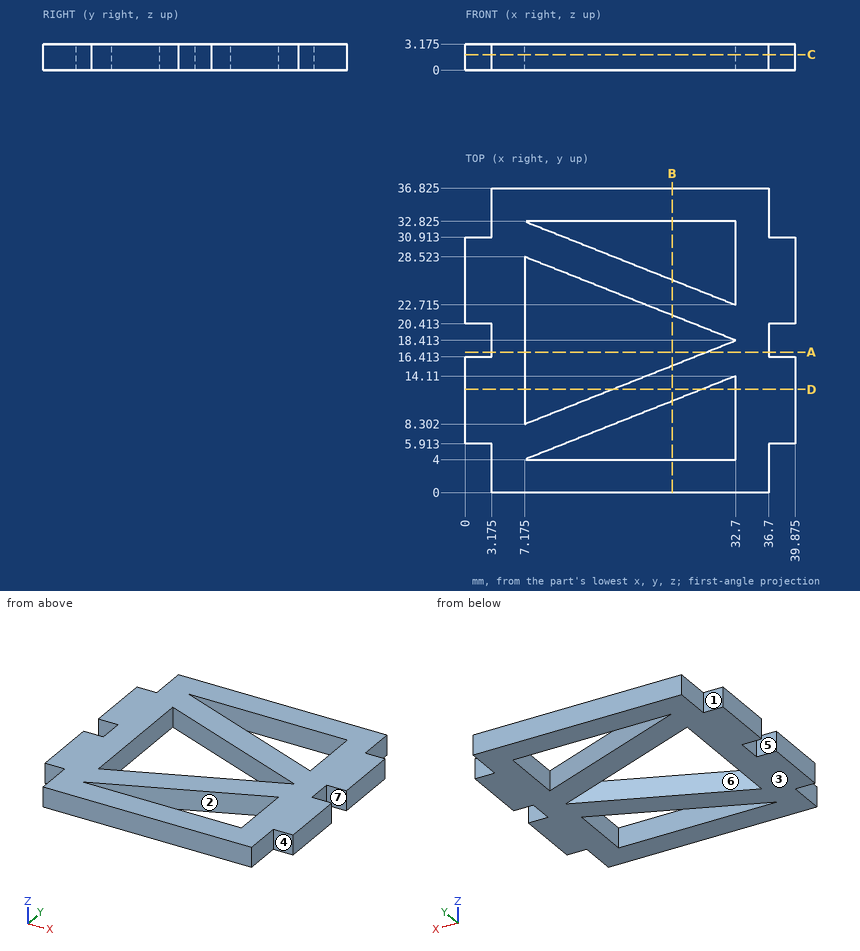
Design review of the part shown in the three views and the two pictorial views. Dimensions are in mm from the part's minimum x, y and z. A direction names the side the tool comes from. Give positions to 0.01 mm unless a question says otherwise; leave off trailing zeros. Loops run counter-clockwise (first coordinate to the right, second up) from the corner with the lowest first, then second, coordinate; pieces in that order, holes last. Notation, with made-up numbers: (1.25, -25) - (42.25, -25) arc R24 ccw to (42.25, -2) - close; hole circle Ø2 at (-22, 11). An arc over 180 degrees is marked (long way). Use CSV: the item, a comma, the result in double quotes. Start each with the question number.
1. Machinability: for the marked faces 4, 5, 6 and 7, which of the approach directions +Z, -Z, +X, -X, +Y, -Y give a long, thin tool a straight path to every point of the face, cutting with its end or side? Answer none if there is none.
2. Add section C-C (z = 1.9). Count the separate pieces of the cut face and the enclosed holes in it.
3. Draft analysis for pull direction Y (two halves, no side actions). For the marked faces 1, 2 and 3, state which applies: released by +Y, released by -Y, zero draft, split by the parting line, or undercut.
4. Add section D-D (y = 12.5). State the section outline as (x, z) points (1 decimal).
5. Wall thickness on L1, parallel to Y at x = 38, z = 1.7; L2, parallel to Y at x = 10, z = 0.4 (1 decimal); L3, parallel to Y at x = 17, z = 1.35 (1 decimal): over which ranges is each line inside the solid? List them lowest first.
6. Insertion check: P1, Ø1.6, axis at x = 38, z = 1, coming from the +Y side; P2, Ø1, axis at x = 1.5, z = 1, coming from the -Y side; P3, Ø1, axis at y = 4, z = 2.5, coming from the +X side. Each pin has a flat end and moves straight along its axis. Give the tip position at first contact, or say it passes through.
7. Add section B-B (x = 25). State the section outline as (y, z) points (1 decimal).
8. Add section A-A (y = 17). State the section outline as (x, z) points (1 decimal).
Results found:
1,face 4,"+Z, -Z, +X, -Y"
1,face 5,"+Z, -Z, -X"
1,face 6,"+Z, -Z"
1,face 7,"+Z, -Z, +X"
2,separate pieces,"1"
2,enclosed holes,"3"
3,face 1,"released by +Y"
3,face 2,"undercut"
3,face 3,"zero draft"
4,outline,"(0, 0) - (7.2, 0) - (7.2, 3.2) - (0, 3.2) - close; (17.8, 0) - (28.6, 0) - (28.6, 3.2) - (17.8, 3.2) - close; (32.7, 0) - (39.9, 0) - (39.9, 3.2) - (32.7, 3.2) - close"
5,L1,"y = 5.91 to 16.41, 20.41 to 30.91"
5,L2,"y = 0 to 4, 5.1 to 9.4, 27.4 to 31.7, 32.8 to 36.8"
5,L3,"y = 0 to 4, 7.9 to 12.2, 24.6 to 28.9, 32.8 to 36.8"
6,P1,"stops at y = 30.91"
6,P2,"stops at y = 5.91"
6,P3,"stops at x = 36.7"
7,outline,"(0, 0) - (4, 0) - (4, 3.2) - (0, 3.2) - close; (11.1, 0) - (15.4, 0) - (15.4, 3.2) - (11.1, 3.2) - close; (21.5, 0) - (25.8, 0) - (25.8, 3.2) - (21.5, 3.2) - close; (32.8, 0) - (36.8, 0) - (36.8, 3.2) - (32.8, 3.2) - close"
8,outline,"(3.2, 0) - (7.2, 0) - (7.2, 3.2) - (3.2, 3.2) - close; (29.1, 0) - (36.7, 0) - (36.7, 3.2) - (29.1, 3.2) - close"
